For this review, use the dimensioned drawing (mm, ordinates from the lowest corner) and the shaded views. A direction names the side the tool comes from. Round coordinates to 2 decimals unless told otherwise and drop trailing zeros. Write each loop counter-clockwise with the first axis right and the second up, starting at its lowest first coordinate (ties: lowest second). Pieces come first, ordered by that corner, then holes. Notation, with made-up numbers: M -16.5,5.25 L 9.5,5.25 A23 cw 9.5,21.25 Z; hole C 24.5,88 d4. An arc over 180 degrees is marked long. One line per question, with ' | ' between items.
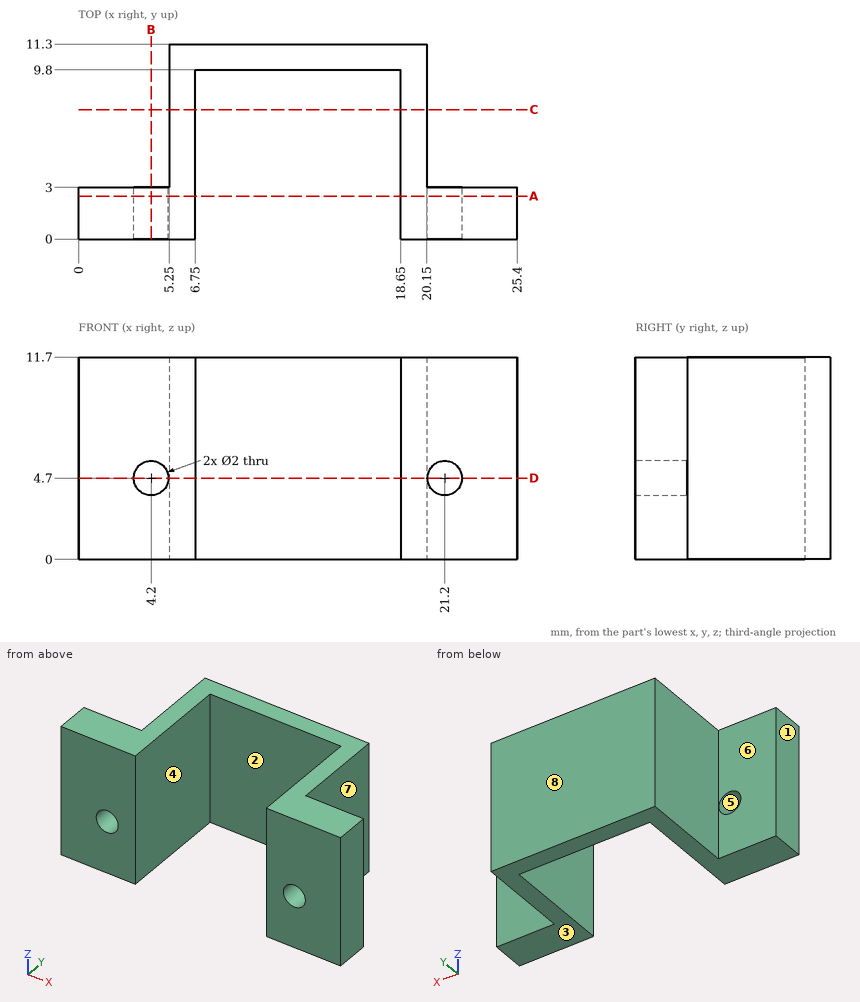
Item 1: Take a section at A-A (y = 2.5). Write out the cut boundary in (x, z), then the cut area to 3 significant figures.
Results:
outline: M 0,0 L 6.75,0 L 6.75,11.7 L 0,11.7 Z; M 18.65,0 L 25.4,0 L 25.4,11.7 L 18.65,11.7 Z; hole C 4.2,4.7 d2; hole C 21.2,4.7 d2 | area: 152 mm2
Item 2: To check wall thickness, follow line 1 along X through (y, z) = (6.75, 5.25); line 2 along X through (y, z) = (1.5, 10.5); line 3 along X through (y, z) = (1.8, 4.7). State the ranges of each line that lie inside material, in increasing order. Write a range as from..to.
Results:
line 1: 5.25..6.75, 18.65..20.15 | line 2: 0..6.75, 18.65..25.4 | line 3: 0..3.2, 5.2..6.75, 18.65..20.2, 22.2..25.4
Item 3: Take a section at B-B (x = 4.2). Write out the cut boundary in (y, z).
Results:
outline: M 0,0 L 3,0 L 3,3.7 L 0,3.7 Z; M 0,5.7 L 3,5.7 L 3,11.7 L 0,11.7 Z
Item 4: Insertion check: pin 1 Ø1.8 at (x, z) = (21.2, 4.7) entering from -Y; pin 2 Ø3 at (y, z) = (5, 6) entering from -X; pin 3 Ø2.5 at (y, z) = (8, 5.5) entering from +X; pin 4 Ø4 at (x, z) = (22.5, 3.5) entering from +Y. Each pin has a flat end and moves straight along its axis. Give the tip position at first contact, or say it passes through.
Results:
pin 1: through | pin 2: x = 5.25 | pin 3: x = 20.15 | pin 4: y = 3
Item 5: Machinability: for the marked faces 4, 5, 6, 7 and 8, which of the approach directions +Z, -Z, +X, -X, +Y, -Y give a long, thin tool a straight path to every point of the face, cutting with its end or side? Answer none if there is none.
Results:
face 4: +Z, -Z, -Y | face 5: +Y, -Y | face 6: +Z, -Z, -X, +Y | face 7: +Z, -Z, +X, +Y | face 8: +Z, -Z, +X, -X, +Y
Item 6: Mouldability with a two-part tool opening along X and no side actions: class the marked faces 1, 2 and 3 as +X half, -X half, draft (parallel to the pull), parting line (faces both ways), or undercut.
Results:
face 1: -X half | face 2: undercut | face 3: draft
Item 7: Take a section at D-D (z = 4.7). Write out the cut boundary in (x, y).
Results:
outline: M 0,0 L 3.2,0 L 3.2,3 L 0,3 Z; M 5.2,0 L 6.75,0 L 6.75,9.8 L 18.65,9.8 L 18.65,0 L 20.2,0 L 20.2,3 L 20.15,3 L 20.15,11.3 L 5.25,11.3 L 5.25,3 L 5.2,3 Z; M 22.2,0 L 25.4,0 L 25.4,3 L 22.2,3 Z
Item 8: Take a section at C-C (y = 7.5). Write out the cut boundary in (x, z), then the cut area to 3 significant figures.
Results:
outline: M 5.25,0 L 6.75,0 L 6.75,11.7 L 5.25,11.7 Z; M 18.65,0 L 20.15,0 L 20.15,11.7 L 18.65,11.7 Z | area: 35.1 mm2
